Geometry: final body of the model. Coordinates: model frame, mm. A direction names the side the tool comes from. Round coordinates to 2 decimals unless told otherwise and drop trailing zeros. Use a Markdown table: item, result. Add a question column.
```python
from build123d import *

# Parameters (mm, degrees)
BOSS_EXTRU_1_DEPTH      = 12.5
BOSS_EXTRU_1_DEPTH_BACK = 2.5
ESQUISSE1_R             = 1
ENL_V_START             = -82.38334833
ENL_V_MAT_EXTRU_1_DEPTH = 82.38334833
ESQUISSE3_R             = 1
ENL_V_MAT_EXTRU_2_DEPTH = 12.5


# Read off the part's stored shape, not the designer's step: Enl_v. mat.-Extru.1
with BuildPart() as part:
    # Esquisse1 → Boss.-Extru.1 (new, two sides: drawn at the far end of the back side and taken through both)
    with BuildSketch(Plane.XY.offset(-BOSS_EXTRU_1_DEPTH_BACK)):
        with BuildLine():
            add(Edge.make_bspline(
                [(-75, -18.910504263), (-56.686373288, -33.096877551), (-10, -18.910504263)],
                knots=[0.563496207, 0.563496207, 0.563496207, 1, 1, 1], degree=2))
            Line((-10, -18.910504263), (8.718662863, -2.287994294))
            Line((8.718662863, -2.287994294), (7.390662863, -0.792529149))
            Line((7.390662863, -0.792529149), (-0.086662863, -7.432529149))
            Line((-0.086662863, -7.432529149), (-2.742662863, -4.441598859))
            Line((-2.742662863, -4.441598859), (4.734662863, 2.198401141))
            Line((4.734662863, 2.198401141), (2.742662863, 4.441598859))
            Line((2.742662863, 4.441598859), (-4.734662863, -2.198401141))
            Line((-4.734662863, -2.198401141), (-7.390662863, 0.792529149))
            Line((-7.390662863, 0.792529149), (5, 11.795661075))
            Line((5, 11.795661075), (5, 60))
            ThreePointArc((5, 60), (0, 65), (-5, 60))
            Line((-5, 60), (-5, 55))
            Line((-5, 55), (-18.333333333, 55))
            Line((-18.333333333, 55), (-18.333333333, 60))
            ThreePointArc((-18.333333333, 60), (-23.333333333, 65), (-28.333333333, 60))
            Line((-28.333333333, 60), (-28.333333333, 55))
            Line((-28.333333333, 55), (-41.666666667, 55))
            Line((-41.666666667, 55), (-41.666666667, 60))
            ThreePointArc((-41.666666667, 60), (-46.666666667, 65), (-51.666666667, 60))
            Line((-51.666666667, 60), (-51.666666667, 55))
            Line((-51.666666667, 55), (-65, 55))
            Line((-65, 55), (-65, 60))
            ThreePointArc((-65, 60), (-70, 65), (-75, 60))
            add(Edge.make_bspline(
                [(-75, 60), (-96.634514155, -1.089766286), (-75, -18.910504263)],
                knots=[0, 0, 0, 0.548330399, 0.548330399, 0.548330399], degree=2))
        make_face()
        with Locations((-23.333333333, 60)):
            Circle(ESQUISSE1_R, mode=Mode.SUBTRACT)
        with Locations((0, 60)):
            Circle(ESQUISSE1_R, mode=Mode.SUBTRACT)
        with Locations((-46.666666667, 60)):
            Circle(ESQUISSE1_R, mode=Mode.SUBTRACT)
        with Locations((-70, 60)):
            Circle(ESQUISSE1_R, mode=Mode.SUBTRACT)
    extrude(amount=BOSS_EXTRU_1_DEPTH + BOSS_EXTRU_1_DEPTH_BACK)

    # Enl_v. mat.-Extru.1 outline → Enl_v. mat.-Extru.1 (cut)
    with BuildSketch(Plane(origin=(5, 0, 0), x_dir=(0, 0, -1), z_dir=(1, 0, 0)).offset(ENL_V_START)):
        Polygon((-10.5, 65.000000033), (-10.5, 53), (-6.5, 53), (-6.5, 65.000000025), align=None)
        Polygon((-3.5, 65.000000025), (-3.5, 53), (0.5, 53), (0.5, 65.000000033), align=None)
    extrude(amount=ENL_V_MAT_EXTRU_1_DEPTH, mode=Mode.SUBTRACT)

    # Esquisse3 → Enl_v. mat.-Extru.2 (cut)
    with BuildSketch(Plane(origin=(4.98, -5.607994294, 0), x_dir=(0.7477325725150671, 0.6640000000000001, 0), z_dir=(0.6640000000000001, -0.7477325725150671, 0))):
        with BuildLine():
            Line((5, 12.5), (-2.5, 12.5))
            ThreePointArc((-2.5, 12.5), (2.803300859, 10.303300859), (5, 5))
            Line((5, 5), (5, 12.5))
        make_face()
        with BuildLine():
            Line((5, -2.5), (5, 5))
            ThreePointArc((5, 5), (2.803300859, -0.303300859), (-2.5, -2.5))
            Line((-2.5, -2.5), (5, -2.5))
        make_face()
        with Locations((-2.5, 5)):
            Circle(ESQUISSE3_R)
    extrude(amount=-ENL_V_MAT_EXTRU_2_DEPTH, mode=Mode.SUBTRACT)


solid = part.part
```
1) Pin query (flat end, axial travel): P1, Ø2, axis at y = 57, z = -1.5, coming from the +X side; P2, Ø6, axis at x = -14.5, z = 1.5, coming from the -Y side; P3, Ø2.5, axis at x = -56.5, z = 5, coming from the +Y side. Return the tip coordinate at first contact, or that it passes through.
2) Set-up query: faces 4 (the flat face through (0.11, -1.91, 4.89)), 5 (the flat face through (-18.333, 57, -2)), 6 (the flat face through (-37, 53, 9)). Return all of +Z, -Z, +X, -X, +Y, -Y with unobstructed straight access to the full face (end or side cutting, diameter ignored); none if empty.
3) Material intervals for L1, parallel to Z at x = -4, y = 53.5; L2, parallel to Y at x = 0, z = -1.4; L3, parallel to X at y = -6, z = 3.5, sorted ascending. Write a range as from..to.
4) Draft query along Z for faces 1 (the flat face through (-5, 58, 11)), 2 (the flat face through (-37, 53, 2)), 3 (the flat face through (-47, 17, -2.5)). Return one class per face: released by +Z, released by -Z, zero draft, split by the parting line, or undercut.
Output values:
| question | item | result |
|---|---|---|
| 1 | P1 | stops at x = 5 |
| 1 | P2 | stops at y = -21.06 |
| 1 | P3 | stops at y = 55 |
| 2 | face 4 | +Z, -Z |
| 2 | face 5 | +Z, -Z, +Y |
| 2 | face 6 | +X, -X, +Y |
| 3 | L1 | z = -2.5..-0.5, 3.5..6.5, 10.5..12.5 |
| 3 | L2 | y = -10.03..-7.36, -2.01..2.01, 7.36..59, 61..65 |
| 3 | L3 | x = -83.57..-1.36, 1.53..4.54 |
| 4 | face 1 | zero draft |
| 4 | face 2 | undercut |
| 4 | face 3 | released by -Z |
